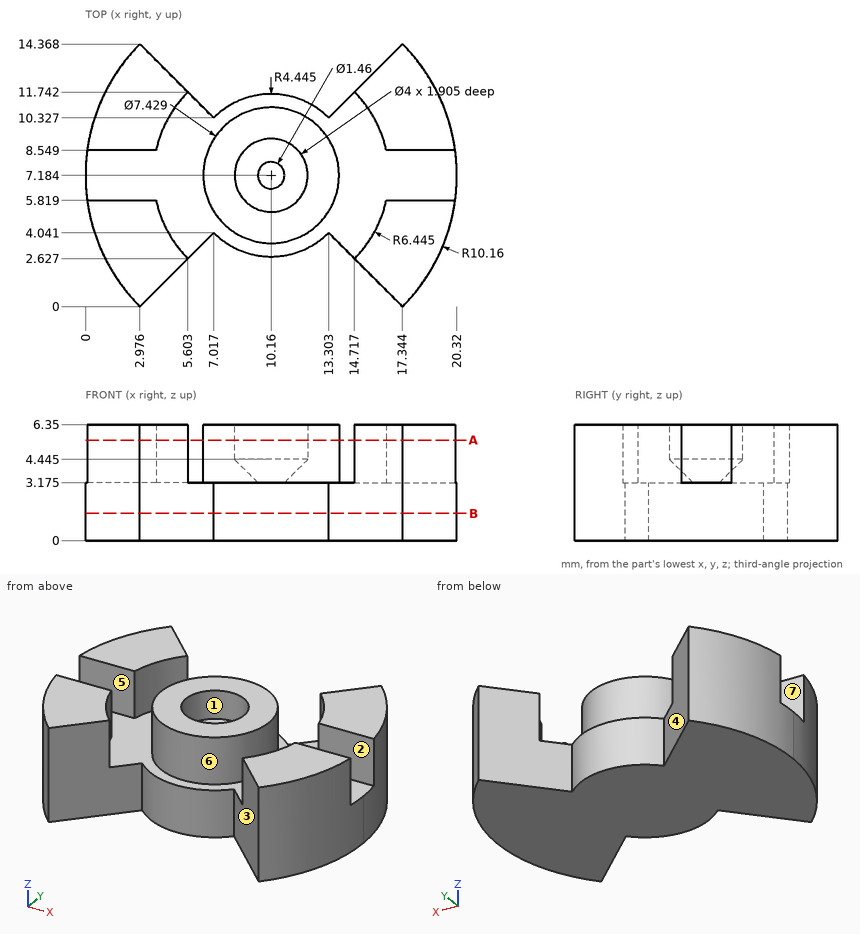
Check sheet for the drawn part. Datum: minimum x, y, z corner. Units: mm. A direction names the side the tool comes from. Round coordinates to 2 decimals unless told otherwise and drop trailing zeros. Loops run counter-clockwise (first coordinate to the right, second up) from the corner with the lowest first, then second, coordinate; pieces in that order, holes last. Notation, with made-up numbers: M 47,-36.75 L 57,-36.75 A20 ccw 57,2.25 Z; hole C -9,86.5 d10. An arc over 180 degrees is marked long. One line per question, with ' | ' between items. Start each with the question number.
Item 1: Release check for a two-part mould opening along X. For the marked faces 6 and 7 record: released by +X, released by -X, zero draft, split by the parting line, or undercut.
Item 2: Gauge pin test, flat ends, axial feed: pin 1 Ø4.5 at (x, y) = (10.16, 7.18) entering from -Z; pin 2 Ø1.6 at (x, y) = (10.5, 7.5) entering from +Z; pin 3 Ø1 at (x, z) = (12, 2) entering from -Y (1 decimal); pin 4 Ø3.5 at (x, z) = (1.5, 5) entering from +Y. Record the tip position at first contact, or that the pin passes through.
Item 3: Section check A-A (z = 5.5). State how many separate pieces and enclosed holes the cut face has, and give its area (3 significant figures).
Item 4: Section check B-B (z = 1.5). Record the boundary of the cut face in (x, y) (1 decimal), and give its area (3 significant figures).
Item 5: Set-up check for the marked faces 1, 2, 3, 4 and 5: record each of +Z, -Z, +X, -X, +Y, -Y from which the full face is reachable in a straight line by a thin tool's end or side.
Item 6: Scan lines: probe 1 along Y at (x, z) = (10.16, 5.7) (1 decimal); probe 2 along Z at (x, y) = (15.75, 9) (1 decimal); probe 3 along X at (y, z) = (8.75, 5) (1 decimal). Record each from-to range of solid material in increasing order.
Worked out:
1) face 6: undercut | face 7: zero draft
2) pin 1: z = 0 | pin 2: z = 3.71 | pin 3: y = 2.9 | pin 4: y = 14.37
3) separate pieces: 5 | enclosed holes: 1 | area: 107 mm^2
4) outline: M 3,0 L 7,4 A4.4 ccw 13.3,4 L 17.3,0 A10.2 ccw 17.3,14.4 L 13.3,10.3 A4.4 ccw 7,10.3 L 3,14.4 A10.2 ccw Z | area: 193 mm^2
5) face 1: +Z | face 2: +Z, +X | face 3: +Z, -Z, -Y | face 4: +Z, -Z, +Y | face 5: +Z, -X
6) probe 1: 3.5 to 5.2, 9.2 to 10.9 | probe 2: 0 to 3.2 | probe 3: 0.1 to 3.9, 6.8 to 8.9, 11.4 to 13.5, 16.4 to 20.2
